from build123d import *

# Parameters (mm, degrees)
SCHIZZO1_W                   = 4
SCHIZZO1_H                   = 4
ESTRUSIONE_ESTRUSIONE1_DEPTH = 4


with BuildPart() as part:
    # Schizzo1 → Estrusione-Estrusione1 (new body)
    with BuildSketch(Plane(origin=(0, 0, 0), x_dir=(1, 0, 0), z_dir=(0, 1, 0))):
        with BuildLine():
            Line((-2, 16), (-16.163229875, 16))
            ThreePointArc((-16.163229875, 16), (-25.984761547, 0.200208393), (-23, -18.162446581))
            Line((-23, -18.162446581), (-23, -6))
            Line((-23, -6), (-9, -6))
            Line((-9, -6), (-9, 3))
            Line((-9, 3), (9, 3))
            Line((9, 3), (9, -6))
            Line((9, -6), (23, -6))
            Line((23, -6), (23, -18.162446581))
            ThreePointArc((23, -18.162446581), (25.984761547, 0.200208393), (16.163229875, 16))
            Line((16.163229875, 16), (2, 16))
            Line((2, 16), (-2, 16))
        make_face()
        with Locations((0, 18)):
            Rectangle(SCHIZZO1_W, SCHIZZO1_H)
    extrude(amount=ESTRUSIONE_ESTRUSIONE1_DEPTH)


solid = part.part
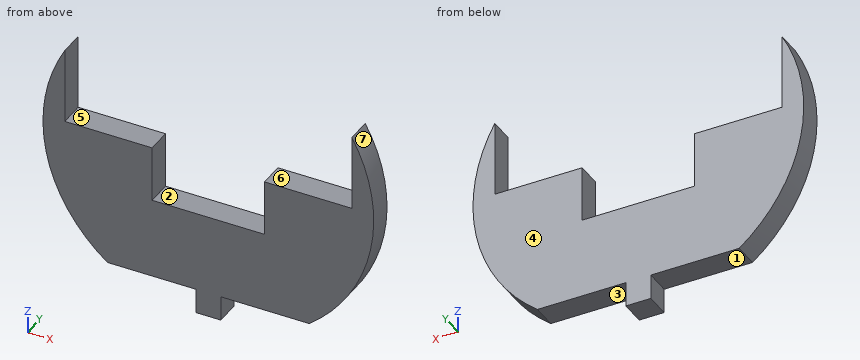
Read the model definition and answer for the solid it produces. Units are mm, in the model's axes. Face numbers are marked on the shaded views. A direction names the side the tool comes from. Coordinates: 2 decimals unless noted, no trailing zeros. Order: outer loops, then holes, each group sorted by start corner. A loop starts at its lowest first (then second) coordinate and runs counter-clockwise, first axis right, second up. Notation, with made-up numbers: (83, 75.5) -> (122, 75.5) arc R7 ccw to (122, 86.5) -> close; hole circle Ø3 at (64, -7.75). An arc over 180 degrees is marked (long way). Answer as a JSON object with one key per item and string values.
1) A tool of negligible diameter and unlimited length cuts with its end or side. For the marked faces 1, 2 and 3, from which of +Z, -Z, +X, -X, +Y, -Y can it reach the whole face along a straight path? Write none if from no direction.
Model answer:
{"face 1": "-Z, -X, +Y, -Y", "face 2": "+Z, +Y, -Y", "face 3": "-Z, +X, +Y, -Y"}
2) A cutting plane is placed at A-A, the plane z = 10. Determine the outline of the cut face in (x, y).
Model answer:
{"outline": "(-26.02, 0) -> (-23, 0) -> (-23, 4) -> (-26.02, 4) -> close; (23, 0) -> (26.02, 0) -> (26.02, 4) -> (23, 4) -> close"}
3) Consider line 1 along Z through (x, y) = (-13.5, 2.15); line 2 along X through (y, z) = (1.25, 9); line 3 along Z through (x, y) = (-0.5, 1.5). Determine where each line is inside the solid, lowest interval first. Write a range as from..to.
Model answer:
{"line 1": "z = -16..6", "line 2": "x = -26.2..-23, 23..26.2", "line 3": "z = -20..-3"}
4) The mould has two halves that part along X. Classify the marked faces 4, 5, 6 and 7: released by +X, released by -X, zero draft, split by the parting line, or undercut.
Model answer:
{"face 4": "zero draft", "face 5": "undercut", "face 6": "undercut", "face 7": "released by +X"}
5) A cutting plane is placed at B-B, the plane y = 1.2. Determine the outline of the cut face in (x, z).
Model answer:
{"outline": "(-23, 6) -> (-23, 18.16) arc R26.5 ccw to (-16.16, -16) -> (-2, -16) -> (-2, -20) -> (2, -20) -> (2, -16) -> (16.16, -16) arc R26.5 ccw to (23, 18.16) -> (23, 6) -> (9, 6) -> (9, -3) -> (-9, -3) -> (-9, 6) -> close"}
6) A cutting plane is placed at D-D, the plane x = -14. Determine the outline of the cut face in (y, z).
Model answer:
{"outline": "(0, -16) -> (4, -16) -> (4, 6) -> (0, 6) -> close"}
7) Each of these flat-tipped pins is pushed along its axis until it touches: pin 1 (1.2 mm diameter, centred on y = 2, z = -18, fed in from -X); pin 2 (1 mm diameter, centred on y = 2, z = 1.5, fed in from -X); pin 3 (1.2 mm diameter, centred on y = 2.5, z = -17.5, fed in from +X). Where does it stop, or does it pass through?
Model answer:
{"pin 1": "stops at x = -2", "pin 2": "stops at x = -26.33", "pin 3": "stops at x = 2"}
8) A cutting plane is placed at C-C, the plane z = 1. Determine the outline of the cut face in (x, y).
Model answer:
{"outline": "(-26.2, 0) -> (-9, 0) -> (-9, 4) -> (-26.2, 4) -> close; (9, 0) -> (26.2, 0) -> (26.2, 4) -> (9, 4) -> close"}
